from build123d import *

# Parameters (mm, degrees)
SKIZZE1_W                       = 8
SKIZZE1_H                       = 75
BASIS_BLECH1_DEPTH              = 2
KANTE_LASCHE3_STRIP_W           = 12
KANTE_LASCHE3_STRIP_H           = 2
KANTE_LASCHE3_STRIP_CUT_DEPTH   = 8
KANTE_LASCHE3_DEPTH             = 8
KANTE_LASCHE4_STRIP_W           = 12
KANTE_LASCHE4_STRIP_H           = 2
KANTE_LASCHE4_STRIP_CUT_DEPTH   = 8
KANTE_LASCHE4_DEPTH             = 8
SCHNITT_LINEAR_AUSTRAGEN1_DEPTH = 2


# Sheet-metal steps are written as plain solids
with BuildPart() as part:
    # Skizze1 → Basis-Blech1 (new body)
    with BuildSketch(Plane.XY):
        with Locations((4, 37.5)):
            Rectangle(SKIZZE1_W, SKIZZE1_H)
    extrude(amount=-BASIS_BLECH1_DEPTH)

    # Kante-Lasche3 strip (across the edge) → Kante-Lasche3 strip cut (cut)
    with BuildSketch(Plane(origin=(0, 75, -2), x_dir=(0, -1, 0), z_dir=(1, 0, 0))):
        with Locations((-4, -1)):
            Rectangle(KANTE_LASCHE3_STRIP_W, KANTE_LASCHE3_STRIP_H)
    kante_lasche3_strip_cut = extrude(amount=KANTE_LASCHE3_STRIP_CUT_DEPTH, mode=Mode.SUBTRACT)

    # Kante-Lasche3 section (across the edge) → Kante-Lasche3 (add)
    with BuildSketch(Plane(origin=(0, 75, -2), x_dir=(0, -1, 0), z_dir=(1, 0, 0))):
        with BuildLine():
            Line((-2, 2), (-2, 38))
            Line((-2, 38), (0, 38))
            Line((0, 38), (0, 2))
            ThreePointArc((0, 2), (0.585786438, 0.585786438), (2, 0))
            Line((2, 0), (2, -2))
            ThreePointArc((2, -2), (-0.828427125, -0.828427125), (-2, 2))
        make_face()
    kante_lasche3 = extrude(amount=KANTE_LASCHE3_DEPTH)

    # Kante-Lasche4 strip (across the edge) → Kante-Lasche4 strip cut (cut)
    with BuildSketch(Plane(origin=(0, 75, -40), x_dir=(0, 0, 1), z_dir=(1, 0, 0))):
        with Locations((-4, -1)):
            Rectangle(KANTE_LASCHE4_STRIP_W, KANTE_LASCHE4_STRIP_H)
    kante_lasche4_strip_cut = extrude(amount=KANTE_LASCHE4_STRIP_CUT_DEPTH, mode=Mode.SUBTRACT)

    # Kante-Lasche4 section (across the edge) → Kante-Lasche4 (add)
    with BuildSketch(Plane(origin=(0, 75, -40), x_dir=(0, 0, 1), z_dir=(1, 0, 0))):
        with BuildLine():
            Line((-2, 2), (-2, 15))
            Line((-2, 15), (0, 15))
            Line((0, 15), (0, 2))
            ThreePointArc((0, 2), (0.585786438, 0.585786438), (2, 0))
            Line((2, 0), (2, -2))
            ThreePointArc((2, -2), (-0.828427125, -0.828427125), (-2, 2))
        make_face()
    kante_lasche4 = extrude(amount=KANTE_LASCHE4_DEPTH)

    # Skizze23 → Schnitt-Linear austragen1 (cut)
    with BuildSketch(Plane(origin=(0, 0, -42), x_dir=(-1, 0, 0), z_dir=(0, 0, -1))):
        with BuildLine():
            Line((-6.25, 65.75), (-6.25, 68.25))
            ThreePointArc((-6.25, 68.25), (-4, 70.5), (-1.75, 68.25))
            Line((-1.75, 68.25), (-1.75, 65.75))
            ThreePointArc((-1.75, 65.75), (-4, 63.5), (-6.25, 65.75))
        make_face()
    schnitt_linear_austragen1 = extrude(amount=-SCHNITT_LINEAR_AUSTRAGEN1_DEPTH, mode=Mode.SUBTRACT)

    # Spiegeln1: Kante-Lasche3 strip cut, Kante-Lasche3, Kante-Lasche4 strip cut, Kante-Lasche4, Schnitt-Linear austragen1 across plane
    add(kante_lasche3_strip_cut.mirror(Plane(origin=(0, 37.5, 0), x_dir=(0, 0, 1), z_dir=(0, -1, 0))), mode=Mode.SUBTRACT)
    add(kante_lasche3.mirror(Plane(origin=(0, 37.5, 0), x_dir=(0, 0, 1), z_dir=(0, -1, 0))))
    add(kante_lasche4_strip_cut.mirror(Plane(origin=(0, 37.5, 0), x_dir=(0, 0, 1), z_dir=(0, -1, 0))), mode=Mode.SUBTRACT)
    add(kante_lasche4.mirror(Plane(origin=(0, 37.5, 0), x_dir=(0, 0, 1), z_dir=(0, -1, 0))))
    add(schnitt_linear_austragen1.mirror(Plane(origin=(0, 37.5, 0), x_dir=(0, 0, 1), z_dir=(0, -1, 0))), mode=Mode.SUBTRACT)


solid = part.part
CAD build for the part. Positions are in the model's coordinates, mm. A direction names the side the tool comes from. Give positions to 0.01 mm unless a question says otherwise; leave off trailing zeros. Write each loop counter-clockwise with the first axis right and the second up, starting at its lowest first coordinate (ties: lowest second). Pieces come first, ordered by that corner, then holes. Notation, with made-up numbers: M -8.75,9.25 L 5.25,9.25 A25 cw 5.25,33.25 Z; hole C 53,12.5 d10. An arc over 180 degrees is marked long. Put each result on its own line as item: value. Start each with the question number.
(1) Probe L1, parallel to Z at x = 1.5, y = 11; L2, parallel to Y at x = 1.5, z = -5; L3, parallel to Z at x = 3.75, y = 67. List the from-to ranges inside material, lowest first.
(2) Band-saw the part on B-B, the plane y = 6. Write the cut outline in (x, z).
(3) Band-saw the part on C-C, the plane x = 4. Write the cut outline in (y, z), and give its area (3 significant figures).
(4) Which spindle directions (+Z, -Z, +X, -X, +Y, -Y) get a long thin tool onto all of the face, cutting with end or side? Do faces 1 (the face through (6.25, 8, -41)), 2 (the face through (1, 8, -42)), 3 (the face through (3.944, 75.797, -1.141)), 4 (the face through (3.94, 0.57, -2.6)), 5 (the face through (4, 60, -41)). Say none if no direction does.
(5) Mould opens along Z. For faces 6 (the face through (1, 67, -42)), 7 (the face through (0, 38, -1)), 8 (the face through (3.94, 74.43, -2.6)) say: +Z half, -Z half, draft (parallel to the pull), parting line (faces both ways), or undercut.
(6) Band-saw the part on A-A, the plane z = -17.5. Write the cut outline in (x, y).
(7) Band-saw the part on D-D, the plane y = 43.5. Write the cut outline in (x, z).
(8) Flat gauge pins, fed straight in: pin 1 Ø1 at (x, y) = (4.5, 29) entering from -Z; pin 2 Ø0.6 at (x, z) = (4.5, -41) entering from -Y. Where does each tip first touch, or does it go through?
Response values:
1. L1: z = -42 to -40, -2 to 0
1. L2: y = -2 to 0, 75 to 77
1. L3: z = -2 to 0
2. outline: M 0,-42 L 1.88,-42 L 1.88,-40 L 0,-40 Z; M 0,-2 L 8,-2 L 8,0 L 0,0 Z; M 6.12,-42 L 8,-42 L 8,-40 L 6.12,-40 Z
3. outline: M -2,-38 A4 ccw 2,-42 L 4.5,-42 L 4.5,-40 L 2,-40 A2 cw 0,-38 L 0,-4 A2 cw 2,-2 L 73,-2 A2 cw 75,-4 L 75,-38 A2 cw 73,-40 L 70.5,-40 L 70.5,-42 L 73,-42 A4 ccw 77,-38 L 77,-4 A4 ccw 73,0 L 2,0 A4 ccw -2,-4 Z; M 11.5,-42 L 15,-42 L 15,-40 L 11.5,-40 Z; M 60,-42 L 63.5,-42 L 63.5,-40 L 60,-40 Z
3. area: 340 mm2
4. face 1: -Z
4. face 2: -Z, +X, -X, +Y, -Y
4. face 3: +Z, +X, -X, +Y
4. face 4: +X, -X
4. face 5: -Z, +X, -X
5. face 6: -Z half
5. face 7: draft
5. face 8: undercut
6. outline: M 0,-2 L 8,-2 L 8,0 L 0,0 Z; M 0,75 L 8,75 L 8,77 L 0,77 Z
7. outline: M 0,-2 L 8,-2 L 8,0 L 0,0 Z
8. pin 1: stops at z = -2
8. pin 2: stops at y = -0.95
